from build123d import *

# Parameters (mm, degrees)
SKETCH_1_W                       = 272
SKETCH_1_H                       = 20
SM_BASE_FLANGE_1_DEPTH           = 1.5
SM_EDGE_FLANGE_1_STRIP_W         = 7.4732
SM_EDGE_FLANGE_1_STRIP_H         = 1.5
SM_EDGE_FLANGE_1_STRIP_CUT_DEPTH = 20
SM_EDGE_FLANGE_1_DEPTH           = 20
SM_EDGE_FLANGE_2_STRIP_W         = 7.4732
SM_EDGE_FLANGE_2_STRIP_H         = 1.5
SM_EDGE_FLANGE_2_STRIP_CUT_DEPTH = 20
SM_EDGE_FLANGE_2_DEPTH           = 20


# Sheet-metal steps are written as plain solids
with BuildPart() as part:
    # Sketch 1 → Базовая кромка1 (new body)
    with BuildSketch(Plane(origin=(0, 0, 0), x_dir=(1, 0, 0), z_dir=(0, 1, 0))):
        with Locations((136, 10)):
            Rectangle(SKETCH_1_W, SKETCH_1_H)
    extrude(amount=-SM_BASE_FLANGE_1_DEPTH)

    # Ребро-кромка1 strip (across the edge) → Ребро-кромка1 strip cut (cut)
    with BuildSketch(Plane.XY.offset(-20)):
        with Locations((-1.5, -0.75)):
            Rectangle(SM_EDGE_FLANGE_1_STRIP_W, SM_EDGE_FLANGE_1_STRIP_H)
    extrude(amount=SM_EDGE_FLANGE_1_STRIP_CUT_DEPTH, mode=Mode.SUBTRACT)

    # Ребро-кромка1 section (across the edge) → Ребро-кромка1 (add)
    with BuildSketch(Plane.XY.offset(-20)):
        with BuildLine():
            Line((0, 0.7366), (0, 33.5))
            Line((0, 33.5), (1.5, 33.5))
            Line((1.5, 33.5), (1.5, 0.7366))
            ThreePointArc((1.5, 0.7366), (1.715745145, 0.215745145), (2.2366, 0))
            Line((2.2366, 0), (2.2366, -1.5))
            ThreePointArc((2.2366, -1.5), (0.655084973, -0.844915027), (0, 0.7366))
        make_face()
    extrude(amount=SM_EDGE_FLANGE_1_DEPTH)

    # Ребро-кромка2 strip (across the edge) → Ребро-кромка2 strip cut (cut)
    with BuildSketch(Plane(origin=(272, 0, 0), x_dir=(-1, 0, 0), z_dir=(0, 0, -1))):
        with Locations((-1.5, -0.75)):
            Rectangle(SM_EDGE_FLANGE_2_STRIP_W, SM_EDGE_FLANGE_2_STRIP_H)
    extrude(amount=SM_EDGE_FLANGE_2_STRIP_CUT_DEPTH, mode=Mode.SUBTRACT)

    # Ребро-кромка2 section (across the edge) → Ребро-кромка2 (add)
    with BuildSketch(Plane(origin=(272, 0, 0), x_dir=(-1, 0, 0), z_dir=(0, 0, -1))):
        with BuildLine():
            Line((0, 0.7366), (0, 33.5))
            Line((0, 33.5), (1.5, 33.5))
            Line((1.5, 33.5), (1.5, 0.7366))
            ThreePointArc((1.5, 0.7366), (1.715745145, 0.215745145), (2.2366, 0))
            Line((2.2366, 0), (2.2366, -1.5))
            ThreePointArc((2.2366, -1.5), (0.655084973, -0.844915027), (0, 0.7366))
        make_face()
    extrude(amount=SM_EDGE_FLANGE_2_DEPTH)


solid = part.part
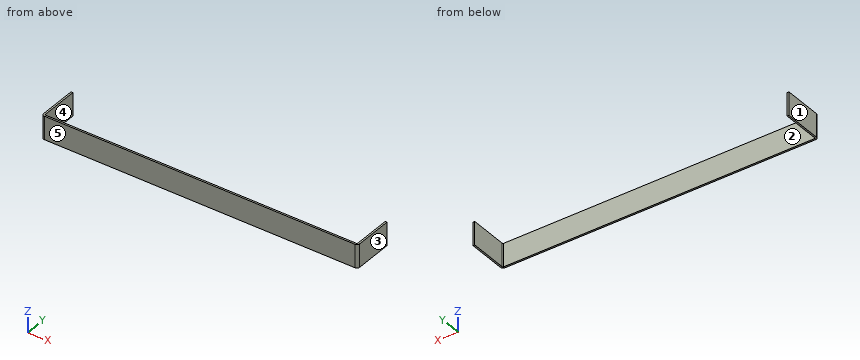
Check sheet for the modelled part. Datum: model origin and axes. Units: mm. Face numbers are marked on the shaded views. A direction names the side the tool comes from. Round coordinates to 2 decimals unless told otherwise and drop trailing zeros. Write each loop counter-clockwise with the first axis right and the second up, starting at its lowest first coordinate (ties: lowest second). Pieces come first, ordered by that corner, then holes. Notation, with made-up numbers: (-3.5, -4) -> (19.5, -4) arc R26 ccw to (19.5, 13) -> close; hole circle Ø4 at (52.5, 22). An arc over 180 degrees is marked (long way). Answer as CSV lines item,"result". Start each with the question number.
1) Section check C-C on x = 238. Enter the section's corners in (y, z).
2) Section check B-B on z = -5. Enter the section's corners in (x, y).
3) Release check for a two-part mould opening along X. For the marked faces 3, 4 and 5 record: pulls with the +X half, pulls with the -X half, needs draft (parallel to the pull), parting line crosses it, or undercut.
4) Go/stop test with a flat-tipped pin: P1, Ø6, axis at x = 200.5, z = -8, coming from the +Y side. Record where the tip stops, or that it passes through.
5) Material ranges on line 1 (X direction, y = 19, z = -14); line 2 (Y direction, x = 212.5, z = -16.75), recorded low to high. Write a range as from..to.
6) Section check A-A on y = 24. Enter the section's corners in (x, z), and give its area (3 significant figures).
7) Tool access check on the marked faces 1 and 2. Record the directions out of +Z, -Z, +X, -X, +Y, -Y that give a thin tool (end or side, any length) a straight path to the whole face; none if there is none.
Found:
1,outline,"(-1.5, -20) -> (0, -20) -> (0, 0) -> (-1.5, 0) -> close"
2,outline,"(0, 0.74) arc R2.24 ccw to (2.24, -1.5) -> (269.76, -1.5) arc R2.24 ccw to (272, 0.74) -> (272, 33.5) -> (270.5, 33.5) -> (270.5, 0.74) arc R0.74 cw to (269.76, 0) -> (2.24, 0) arc R0.74 cw to (1.5, 0.74) -> (1.5, 33.5) -> (0, 33.5) -> close"
3,face 3,"pulls with the +X half"
3,face 4,"undercut"
3,face 5,"needs draft"
4,P1,"stops at y = 0"
5,line 1,"x = 0..1.5, 270.5..272"
5,line 2,"y = -1.5..0"
6,outline,"(0, -20) -> (1.5, -20) -> (1.5, 0) -> (0, 0) -> close; (270.5, -20) -> (272, -20) -> (272, 0) -> (270.5, 0) -> close"
6,area,"60.0 mm^2"
7,face 1,"+Z, -Z, -X, +Y, -Y"
7,face 2,"+Z, -Z, +Y"
